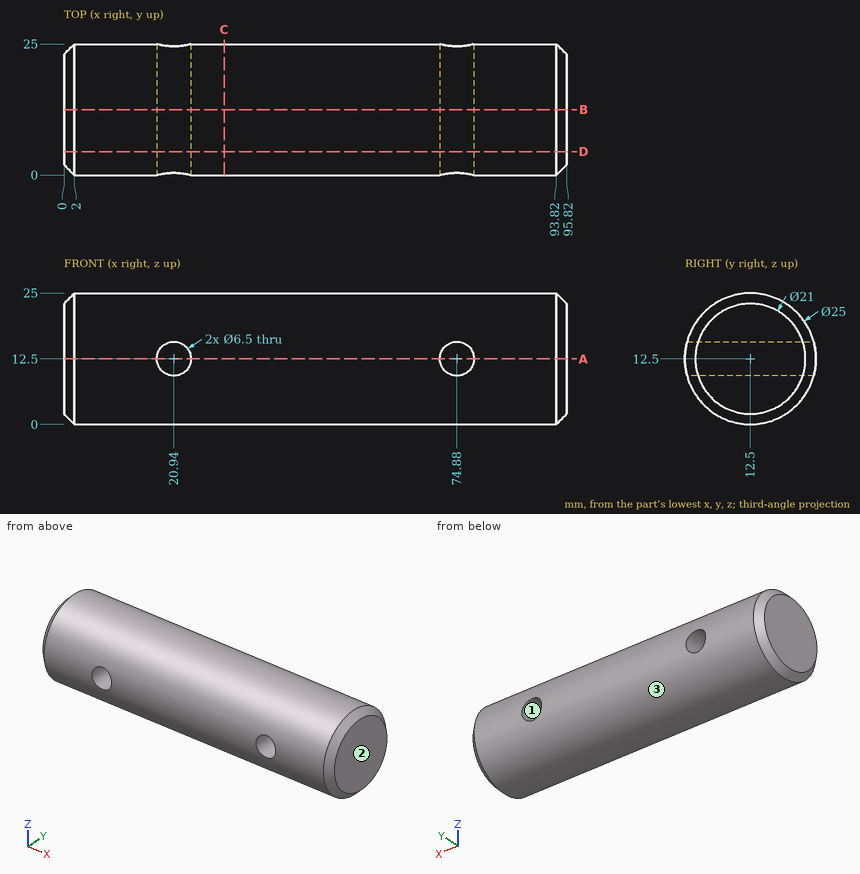
Could you check a few things on this drawing? It's one solid part, dimensions in mm from its lowest x, y, z. Coordinates: 2 decimals unless noted, no trailing zeros. Order: outer loops, then holes, each group sorted by start corner. A loop starts at its lowest first (then second) coordinate and runs counter-clockwise, first axis right, second up.
1) I need wall thicknesses on line 1 (X direction, y = 15, z = 12.5); line 2 (Z direction, x = 35.5, y = 5.75); line 3 (Y direction, x = 68, z = 12.75). Which ranges of each line are inside material? Lowest first, please.
2) We'd pull the mould along Z, two halves only. Please class the marked faces 1, 2 and 3: +Z half, -Z half, draft (parallel to the pull), parting line (faces both ways), or undercut.
3) Imagine slicing it at C-C on x = 30.5. List the corners of the cut face in (y, z) for me, and give its area (3 significant figures).
4) Imagine slicing it at A-A on z = 12.5. List the corners of the cut face in (x, y) for me.
5) Imagine slicing it at D-D on y = 4.5. State how many separate pieces and enclosed holes the cut face has, and give its area (3 significant figures).
6) Will these pins go through, and if not, where does the flat tip stop? pin 1 (4 mm diameter, centred on x = 74.88, z = 12.5, fed in from +Y); pin 2 (2 mm diameter, centred on y = 6.5, z = 17, fed in from -X); pin 3 (4 mm diameter, centred on x = 48, y = 22, fed in from -Z); pin 4 (5 mm diameter, centred on x = 34.5, y = 4.5, fed in from +Z) (3 decimals).
7) Imagine slicing it at B-B on y = 12.5. List the corners of the cut face in (x, z) for me, and give its area (3 significant figures).
Response values:
1. line 1: x = 0 to 17.69, 24.19 to 71.63, 78.13 to 95.82
1. line 2: z = 1.98 to 23.02
1. line 3: y = 0 to 25
2. face 1: undercut
2. face 2: draft
2. face 3: parting line
3. outline: circle Ø25 at (12.5, 12.5)
3. area: 491 mm2
4. outline: (0, 2) - (2, 0) - (17.69, 0) - (17.69, 25) - (2, 25) - (0, 23) - close; (24.19, 0) - (71.63, 0) - (71.63, 25) - (24.19, 25) - close; (78.13, 0) - (93.82, 0) - (95.82, 2) - (95.82, 23) - (93.82, 25) - (78.13, 25) - close
5. separate pieces: 1
5. enclosed holes: 2
5. area: 1,760 mm2
6. pin 1: passes through
6. pin 2: stops at x = 0
6. pin 3: stops at z = 2.5
6. pin 4: stops at z = 23.725
7. outline: (0, 2) - (2, 0) - (93.82, 0) - (95.82, 2) - (95.82, 23) - (93.82, 25) - (2, 25) - (0, 23) - close; hole circle Ø6.5 at (20.94, 12.5); hole circle Ø6.5 at (74.88, 12.5)
7. area: 2,320 mm2
